Source: three-view drawing plus pictorial views. Frame: mm from the lowest corner of the part. Coordinates: 2 decimals unless noted, no trailing zeros. Write each loop counter-clockwise with the first axis right and the second up, starting at its lowest first coordinate (ties: lowest second). Pieces come first, ordered by that corner, then holes. Notation, with made-up numbers: (31.25, 23.25) -> (87.25, 23.25) arc R17 ccw to (87.25, 32.25) -> close; hole circle Ø1 at (7, 81.5). An arc over 180 degrees is marked (long way). One line per item, written item: value.
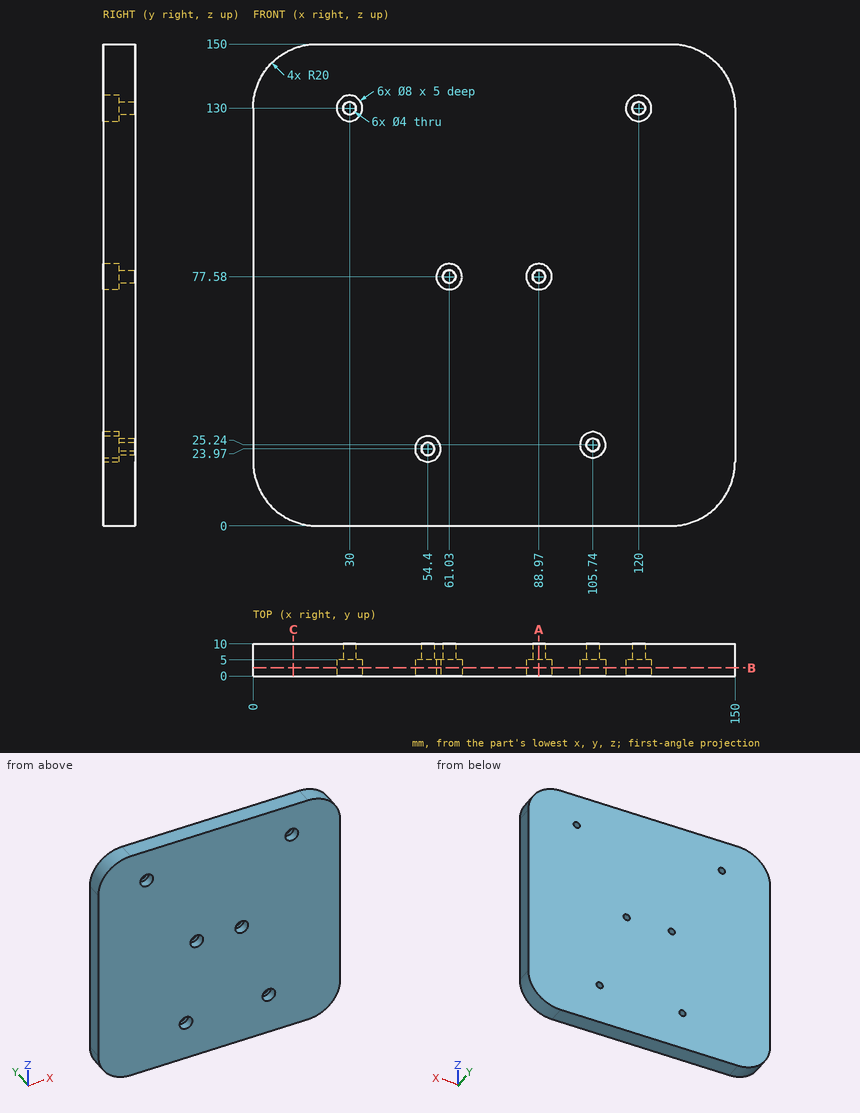
(1) Section A-A (x = 88.97). Return the cut outline in (y, z), then the cut area to 3 significant figures.
Responses:
outline: (0, 0) -> (10, 0) -> (10, 75.58) -> (5, 75.58) -> (5, 73.58) -> (0, 73.58) -> close; (0, 81.58) -> (5, 81.58) -> (5, 79.58) -> (10, 79.58) -> (10, 150) -> (0, 150) -> close
area: 1,440 mm2
(2) Line query: line 1 (X direction, y = 1.8, z = 130); line 2 (X direction, y = 6.2, z = 77.58); line 3 (X direction, y = 4, z = 19.5). Output: solid intervals per line, ascending. Write a range as [from, to].
Responses:
line 1: x = [0, 26], [34, 116], [124, 150]
line 2: x = [0, 59.03], [63.03, 86.97], [90.97, 150]
line 3: x = [0.01, 149.99]
(3) First-contact query: pin 1 (2.5 mm diameter, centred on x = 61, z = 76, fed in from -Y); pin 2 (3.5 mm diameter, centred on x = 88.97, z = 77.58, fed in from -Y). Flat tips, straight axial feed; report the tip coordinate or a pass-through.
Responses:
pin 1: stops at y = 5
pin 2: passes through
(4) Section C-C (x = 12.5). Return the cut outline in (y, z), then the cut area to 3 significant figures.
Responses:
outline: (0, 1.46) -> (10, 1.46) -> (10, 148.54) -> (0, 148.54) -> close
area: 1,470 mm2
(5) Section B-B (y = 2.5). Return the cut outline in (x, z), then the cut area to 3 significant figures.
Responses:
outline: (0, 20) arc R20 ccw to (20, 0) -> (130, 0) arc R20 ccw to (150, 20) -> (150, 130) arc R20 ccw to (130, 150) -> (20, 150) arc R20 ccw to (0, 130) -> close; hole circle Ø8 at (30, 130); hole circle Ø8 at (54.4, 23.97); hole circle Ø8 at (61.03, 77.58); hole circle Ø8 at (88.97, 77.58); hole circle Ø8 at (105.74, 25.24); hole circle Ø8 at (120, 130)
area: 21,900 mm2
